Verification items for the finished model (mm, model axes). Face numbers are marked on the shaded views. A direction names the side the tool comes from. Round coordinates to 2 decimals unless told otherwise and drop trailing zeros. Write each loop counter-clockwise with the first axis right and the second up, starting at its lowest first coordinate (ties: lowest second). Pieces come first, ordered by that corner, then holes.
from build123d import *

# Parameters (mm, degrees)
BOSS_EXTRUDE1_DEPTH = 75
SHELL13_T           = -10
FILLET5_R           = 10
FILLET8_R           = 2
FILLET9_R           = 10


with BuildPart() as part:
    # Sketch1 → Boss-Extrude1 (new body)
    with BuildSketch(Plane(origin=(0, 0, 0), x_dir=(1, 0, 0), z_dir=(0, 1, 0))):
        Polygon((-116.60063424078889, 55.81031027640047), (116.00742939980823, 55.81031027640047), (116.00742939980825, -61.81321623229694), (-116.60063424078888, -61.81321623229694), align=None)
    extrude(amount=BOSS_EXTRUDE1_DEPTH)

    # Shell13
    shell13_openings = [part.faces().sort_by_distance(p)[0] for p in [
        (-0.29660242, 75, 3.001452978),
    ]]
    offset(amount=SHELL13_T, openings=shell13_openings, kind=Kind.INTERSECTION)

    # Fillet5
    fillet5_edges = [part.edges().sort_by_distance(p)[0] for p in [
        (-106.60063424078889, 42.5, -45.81031027640047),
        (-106.60063424078889, 42.5, 51.81321623229694),
        (106.00742939980825, 42.5, 51.81321623229694),
        (106.00742939980823, 42.5, -45.81031027640047),
    ]]
    fillet(fillet5_edges, radius=FILLET5_R)

    # Fillet8
    fillet8_edges = [part.edges().sort_by_distance(p)[0] for p in [
        (116.00742939980825, 75, 3.001452977948233),
        (-0.2966024204903306, 75, -55.81031027640047),
        (-116.60063424078888, 75, 3.001452977948233),
        (-0.2966024204903164, 75, 61.81321623229694),
    ]]
    fillet(fillet8_edges, radius=FILLET8_R)

    # Fillet9
    # the kernel refuses this fillet: 10 mm, written as the material it takes off along each edge
    with BuildSketch(Plane(origin=(106.00742939980825, 75, 51.81321623229694), x_dir=(0, 0, 1), z_dir=(-1, 0, 0))) as fillet9_piece_1:
        with BuildLine():
            CenterArc((8, -2), 2, 0, 90)
            Line((10, -2), (10, 0))
            Line((10, 0), (8, 0))
        make_face()
    revolve(axis=Axis((106.00742939980825, 75, 51.81321623229694), (0, 1, 0)), revolution_arc=90.00000000000001, mode=Mode.SUBTRACT)
    with BuildSketch(Plane(origin=(-106.60063424078888, 75, 51.81321623229694), x_dir=(-1, 0, 1.2e-16), z_dir=(-1.2e-16, 0, -1))) as fillet9_piece_2:
        with BuildLine():
            CenterArc((8, -2), 2, 0, 90)
            Line((10, -2), (10, 0))
            Line((10, 0), (8, 0))
        make_face()
    revolve(axis=Axis((-106.60063424078888, 75, 51.81321623229694), (0, 1, 0)), revolution_arc=90, mode=Mode.SUBTRACT)
    with BuildSketch(Plane(origin=(106.00742939980823, 75, -45.81031027640047), x_dir=(1, 0, -1.2e-16), z_dir=(1.2e-16, 0, 1))) as fillet9_piece_3:
        with BuildLine():
            CenterArc((8, -2), 2, 0, 90)
            Line((10, -2), (10, 0))
            Line((10, 0), (8, 0))
        make_face()
    revolve(axis=Axis((106.00742939980823, 75, -45.81031027640047), (0, 1, 0)), revolution_arc=90, mode=Mode.SUBTRACT)
    with BuildSketch(Plane(origin=(-106.60063424078889, 75, -45.81031027640047), x_dir=(0, 0, -1), z_dir=(1, 0, 0))) as fillet9_piece_4:
        with BuildLine():
            CenterArc((8, -2), 2, 0, 90)
            Line((10, -2), (10, 0))
            Line((10, 0), (8, 0))
        make_face()
    revolve(axis=Axis((-106.60063424078889, 75, -45.81031027640047), (0, 1, 0)), revolution_arc=90.00000000000001, mode=Mode.SUBTRACT)
    with BuildSketch(Plane(origin=(-116.60063424078889, -25, -55.81031027640047), x_dir=(1, 0, 0), z_dir=(0, 1, 0)), Plane(origin=(116.00742939980823, -25, -55.81031027640047), x_dir=(0, 0, 1), z_dir=(0, 1, 0))) as fillet9_piece_5:
        with BuildLine():
            CenterArc((FILLET9_R, -FILLET9_R), FILLET9_R, 90, 90)
            Line((0, -FILLET9_R), (0, 0))
            Line((0, 0), (FILLET9_R, 0))
        make_face()
    extrude(amount=100.00000000000001, mode=Mode.SUBTRACT)
    with BuildSketch(Plane(origin=(-116.60063424078888, -25, 61.81321623229694), x_dir=(1, 0, 0), z_dir=(0, 1, 0)), Plane(origin=(116.00742939980825, -25, 61.81321623229694), x_dir=(0, 0, -1), z_dir=(0, 1, 0))) as fillet9_piece_6:
        with BuildLine():
            CenterArc((FILLET9_R, FILLET9_R), FILLET9_R, 180, 90)
            Line((0, FILLET9_R), (0, 0))
            Line((0, 0), (FILLET9_R, 0))
        make_face()
    extrude(amount=100.00000000000001, mode=Mode.SUBTRACT)


solid = part.part
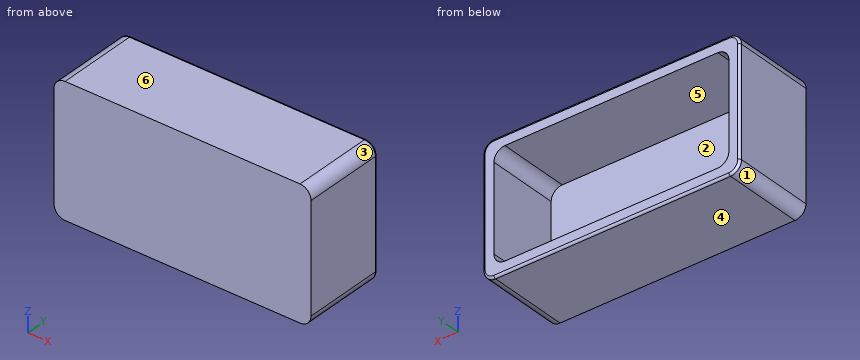
Q1. Sectioned sample at A-A (y = 54). Enter the section's corners in (x, z), plus the area to 3 significant figures.
Recorded:
outline: (-116.6, -45.81) arc R10 ccw to (-106.6, -55.81) - (106.01, -55.81) arc R10 ccw to (116.01, -45.81) - (116.01, 51.81) arc R10 ccw to (106.01, 61.81) - (-106.6, 61.81) arc R10 ccw to (-116.6, 51.81) - close; hole (-106.6, -35.81) arc R10 ccw to (-96.6, -45.81) - (96.01, -45.81) arc R10 ccw to (106.01, -35.81) - (106.01, 41.81) arc R10 ccw to (96.01, 51.81) - (-96.6, 51.81) arc R10 ccw to (-106.6, 41.81) - close
area: 6,600 mm2
Q2. Tool access check on the marked faces 5 and 6. Record the directions out of +Z, -Z, +X, -X, +Y, -Y that give a thin tool (end or side, any length) a straight path to the whole face; none if there is none.
Recorded:
face 5: +Y
face 6: +Z, +X, -X, +Y, -Y
Q3. Depth check by flat-ended pin: P1, Ø3, axis at x = 37, z = 26.5, coming from the +Y side; P2, Ø6, axis at x = 86, z = -8.5, coming from the -Y side. Enter the tip coordinate at first touch or a pass-through.
Recorded:
P1: stops at y = 10
P2: stops at y = 0
Q4. Material ranges on line 1 along Z through (x, y) = (41, 27); line 2 along X through (y, z) = (31, 32.5); line 3 along Y through (x, z) = (51.5, 24.5), recorded low to high.
Recorded:
line 1: z = -55.81 to -45.81, 51.81 to 61.81
line 2: x = -116.6 to -106.6, 106.01 to 116.01
line 3: y = 0 to 10
Q5. Release check for a two-part mould opening along X. For the marked faces 1, 2, 3 and 4 record: released by +X, released by -X, zero draft, split by the parting line, or undercut.
Recorded:
face 1: released by -X
face 2: undercut
face 3: released by +X
face 4: zero draft
Q6. Sectioned sample at B-B (x = -51). Enter the section's corners in (y, z).
Recorded:
outline: (0, -55.81) - (73, -55.81) arc R2 ccw to (75, -53.81) - (75, -45.81) - (10, -45.81) - (10, 51.81) - (75, 51.81) - (75, 59.81) arc R2 ccw to (73, 61.81) - (0, 61.81) - close
Q7. Sectioned sample at C-C (z = 23). Enter the section's corners in (x, y).
Recorded:
outline: (-116.6, 0) - (116.01, 0) - (116.01, 73) arc R2 ccw to (114.01, 75) - (106.01, 75) - (106.01, 10) - (-106.6, 10) - (-106.6, 75) - (-114.6, 75) arc R2 ccw to (-116.6, 73) - close
